The drawing under review shows one solid part. Ordinate dimensions are in mm from its lowest x, y, z. A direction names the side the tool comes from. Coordinates: 2 decimals unless noted, no trailing zeros. Write each loop counter-clockwise with the first axis right and the second up, starting at its lowest first coordinate (ties: lowest second). Pieces come first, ordered by that corner, then holes.
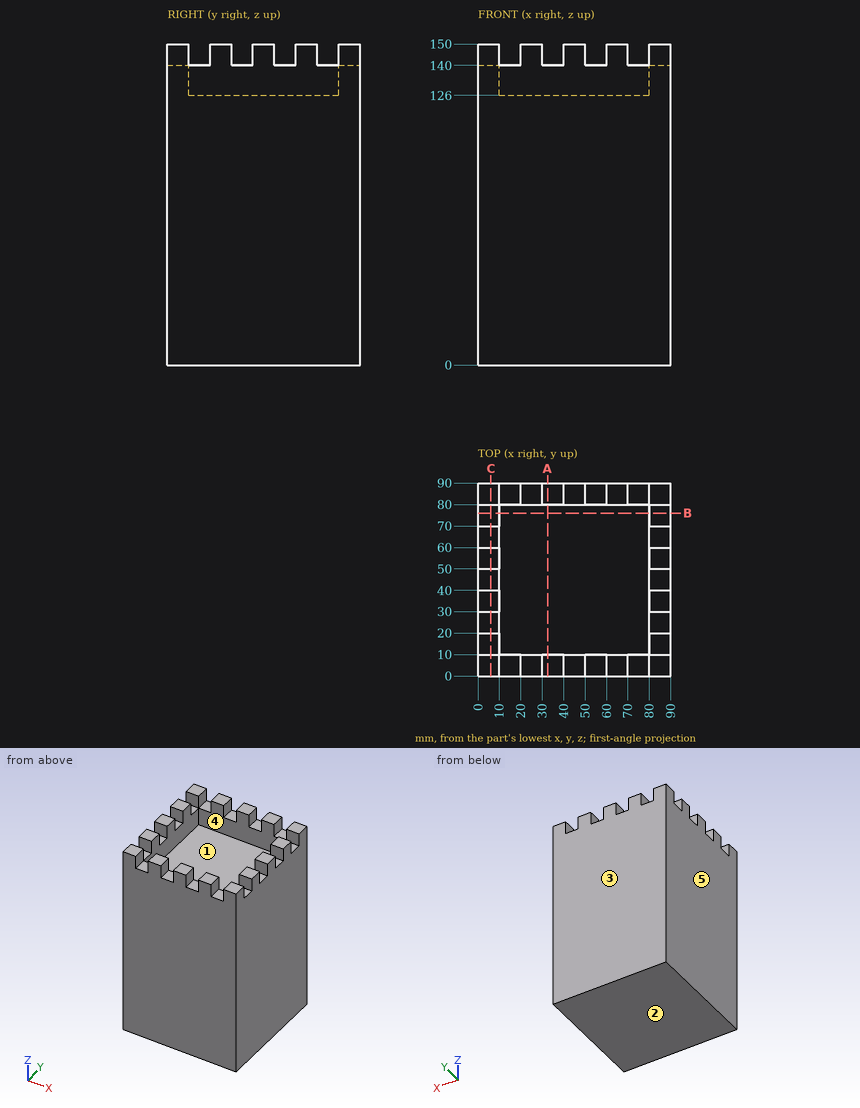
Q1. Clearance check with flat-ended pins moving along their axes: pin 1 Ø3 at (x, y) = (5, 34.5) entering from +Z; pin 2 Ø5 at (x, y) = (66, 62) entering from +Z. State where each tip first meets the part, or that it passes through.
Ans:
pin 1: stops at z = 140
pin 2: stops at z = 126
Q2. Tool access review of the marked faces 4 and 5: name each direction out of +Z, -Z, +X, -X, +Y, -Y from which nothing blocks a thin tool from reaching the whole face with its end or side.
Ans:
face 4: +Z
face 5: +Z, -Z, -X, +Y, -Y
Q3. For probe 1 along X at (y, z) = (30.5, 128.5); probe 2 along Z at (x, y) = (50, 53), list the stretches that pass through material, from the lowest coordinate up.
Ans:
probe 1: x = 0 to 10, 80 to 90
probe 2: z = 0 to 126
Q4. Add section C-C (x = 6). State the section outline as (y, z) points, then the cut area to 3 significant figures.
Ans:
outline: (0, 0) - (90, 0) - (90, 150) - (80, 150) - (80, 140) - (70, 140) - (70, 150) - (60, 150) - (60, 140) - (50, 140) - (50, 150) - (40, 150) - (40, 140) - (30, 140) - (30, 150) - (20, 150) - (20, 140) - (10, 140) - (10, 150) - (0, 150) - close
area: 13,100 mm2
Q5. Draft analysis for pull direction Y (two halves, no side actions). For the marked faces 1, 2 and 3, state which applies: +Y half, -Y half, draft (parallel to the pull), parting line (faces both ways), or undercut.
Ans:
face 1: undercut
face 2: draft
face 3: +Y half
Q6. Add section A-A (x = 32.5). State the section outline as (y, z) points.
Ans:
outline: (0, 0) - (90, 0) - (90, 140) - (80, 140) - (80, 126) - (10, 126) - (10, 140) - (0, 140) - close
